```python
from build123d import *

# Parameters (mm, degrees)
F0_W      = 124.8
F0_H      = 81
F1_DEPTH  = 15.39
F2_W      = 120.8
F2_H      = 77
F3_DEPTH  = 13.39
F4_W      = 124.8
F4_H      = 3
F5_DEPTH  = 1.15
F6_W      = 124.8
F6_H      = 3
F7_DEPTH  = 1.15
F8_W      = 78.7
F8_H      = 3
F9_DEPTH  = 1.15
F10_W     = 78.7
F10_H     = 3
F11_DEPTH = 1.15
F12_W     = 10
F12_H     = 10
F13_DEPTH = 11.82
F14_W     = 10
F14_H     = 10
F15_DEPTH = 11.82
F16_W     = 10
F16_H     = 10
F17_DEPTH = 11.82
F18_W     = 10
F18_H     = 10
F19_DEPTH = 11.82
F20_R     = 1.5
F21_DEPTH = 11.82
F22_R     = 1.5
F23_DEPTH = 11.82
F24_R     = 1.5
F25_DEPTH = 11.82
F26_R     = 1.5
F27_DEPTH = 11.82
F28_W     = 26
F28_H     = 45
F29_DEPTH = 2.001
F30_W     = 12.8
F30_H     = 30.7
F31_DEPTH = 2.001
F32_W     = 17
F32_H     = 12.8
F33_DEPTH = 2.001
F34_R     = 3
F35_DEPTH = 3.3


with BuildPart() as f1:
    # F0 (on Top) → F1 (new body)
    with BuildSketch(Plane.XY):
        Rectangle(F0_W, F0_H)
    extrude(amount=F1_DEPTH)

    # F2 (on face) → F3 (cut)
    with BuildSketch(Plane.XY.offset(15.39)):
        Rectangle(F2_W, F2_H)
    extrude(amount=-F3_DEPTH, mode=Mode.SUBTRACT)

    # F4 (on face) → F5 (cut)
    with BuildSketch(Plane(origin=(0, 40.5, 0), x_dir=(-1, 0, 0), z_dir=(0, 1, 0))):
        with Locations((0, 13.89)):
            Rectangle(F4_W, F4_H)
    extrude(amount=-F5_DEPTH, mode=Mode.SUBTRACT)

    # F6 (on face) → F7 (cut)
    with BuildSketch(Plane.XZ.offset(40.5)):
        with Locations((0, 13.89)):
            Rectangle(F6_W, F6_H)
    extrude(amount=-F7_DEPTH, mode=Mode.SUBTRACT)

    # F8 (on face) → F9 (cut)
    with BuildSketch(Plane(origin=(-62.4, 0, 0), x_dir=(0, -1, 0), z_dir=(-1, 0, 0))):
        with Locations((0, 13.89)):
            Rectangle(F8_W, F8_H)
    extrude(amount=-F9_DEPTH, mode=Mode.SUBTRACT)

    # F10 (on face) → F11 (cut)
    with BuildSketch(Plane.YZ.offset(62.4)):
        with Locations((0, 13.89)):
            Rectangle(F10_W, F10_H)
    extrude(amount=-F11_DEPTH, mode=Mode.SUBTRACT)

    # F12 (on face) → F13 (join)
    with BuildSketch(Plane.XY.offset(2)):
        with Locations((-55.4, 33.5)):
            Rectangle(F12_W, F12_H)
    extrude(amount=F13_DEPTH)

    # F14 (on face) → F15 (join)
    with BuildSketch(Plane.XY.offset(2)):
        with Locations((-55.4, -33.5)):
            Rectangle(F14_W, F14_H)
    extrude(amount=F15_DEPTH)

    # F16 (on face) → F17 (join)
    with BuildSketch(Plane.XY.offset(2)):
        with Locations((55.4, -33.5)):
            Rectangle(F16_W, F16_H)
    extrude(amount=F17_DEPTH)

    # F18 (on face) → F19 (join)
    with BuildSketch(Plane.XY.offset(2)):
        with Locations((55.4, 33.5)):
            Rectangle(F18_W, F18_H)
    extrude(amount=F19_DEPTH)

    # F20 (on face) → F21 (cut)
    with BuildSketch(Plane.XY.offset(13.82)):
        with Locations((-55, 33.5)):
            Circle(F20_R)
    extrude(amount=-F21_DEPTH, mode=Mode.SUBTRACT)

    # F22 (on face) → F23 (cut)
    with BuildSketch(Plane.XY.offset(13.82)):
        with Locations((-55, -33.5)):
            Circle(F22_R)
    extrude(amount=-F23_DEPTH, mode=Mode.SUBTRACT)

    # F24 (on face) → F25 (cut)
    with BuildSketch(Plane.XY.offset(13.82)):
        with Locations((55, -33.5)):
            Circle(F24_R)
    extrude(amount=-F25_DEPTH, mode=Mode.SUBTRACT)

    # F26 (on face) → F27 (cut)
    with BuildSketch(Plane.XY.offset(13.82)):
        with Locations((55, 33.5)):
            Circle(F26_R)
    extrude(amount=-F27_DEPTH, mode=Mode.SUBTRACT)

    # F28 (on face) → F29 (cut, through all)
    with BuildSketch(Plane.XY.offset(2)):
        with Locations((44.4, 5)):
            Rectangle(F28_W, F28_H)
    extrude(amount=-F29_DEPTH, mode=Mode.SUBTRACT)

    # F30 (on face) → F31 (cut, through all)
    with BuildSketch(Plane.XY.offset(2)):
        with Locations((9.5, 0)):
            Rectangle(F30_W, F30_H)
    extrude(amount=-F31_DEPTH, mode=Mode.SUBTRACT)

    # F32 (on face) → F33 (cut, through all)
    with BuildSketch(Plane.XY.offset(2)):
        with Locations((24.9, -29.1)):
            Rectangle(F32_W, F32_H)
    extrude(amount=-F33_DEPTH, mode=Mode.SUBTRACT)

    # F34 (on face) → F35 (join)
    with BuildSketch(Plane.XY.offset(2)):
        with Locations((24.4, 13.2)):
            Circle(F34_R)
        with Locations((24.4, -15.8)):
            Circle(F34_R)
        with Locations((-34.6, 13.2)):
            Circle(F34_R)
        with Locations((-34.6, -15.8)):
            Circle(F34_R)
    extrude(amount=F35_DEPTH)


solid = f1.part
```
Source: CAD feature listing. Evaluate the final solid. Frame: model axes, mm. A direction names the side the tool comes from. Round coordinates to 2 decimals unless told otherwise and drop trailing zeros. Loops run counter-clockwise (first coordinate to the right, second up) from the corner with the lowest first, then second, coordinate; pieces in that order, holes last.
(1) Section query D-D (y = -3). Output: boundary loops of the cut face in (x, z).
From the geometry:
outline: (-62.4, 0) - (3.1, 0) - (3.1, 2) - (-60.4, 2) - (-60.4, 15.39) - (-61.25, 15.39) - (-61.25, 12.39) - (-62.4, 12.39) - close; (15.9, 0) - (31.4, 0) - (31.4, 2) - (15.9, 2) - close; (57.4, 0) - (62.4, 0) - (62.4, 12.39) - (61.25, 12.39) - (61.25, 15.39) - (60.4, 15.39) - (60.4, 2) - (57.4, 2) - close
(2) Pull-direction query (Y, two-part tool) for faces 3 (the flat face through (1, 39.35, 14)), 4 (the flat face through (56, -32, 13.82)), 5 (the flat face through (61.25, -1, 14)); classes: +Y half, -Y half, draft (parallel to the pull), parting line (faces both ways), or undercut.
From the geometry:
face 3: +Y half
face 4: undercut
face 5: draft
(3) Section query C-C (z = 9). Output: boundary loops of the cut face in (x, y), and give its area (3 significant figures).
From the geometry:
outline: (-62.4, -40.5) - (62.4, -40.5) - (62.4, 40.5) - (-62.4, 40.5) - close; hole (-60.4, -28.5) - (-50.4, -28.5) - (-50.4, -38.5) - (50.4, -38.5) - (50.4, -28.5) - (60.4, -28.5) - (60.4, 28.5) - (50.4, 28.5) - (50.4, 38.5) - (-50.4, 38.5) - (-50.4, 28.5) - (-60.4, 28.5) - close; hole circle Ø3 at (-55, -33.5); hole circle Ø3 at (-55, 33.5); hole circle Ø3 at (55, -33.5); hole circle Ø3 at (55, 33.5)
area: 1,180 mm2
(4) Section query A-A (y = 21). Output: boundary loops of the cut face in (x, z).
From the geometry:
outline: (-62.4, 0) - (31.4, 0) - (31.4, 2) - (-60.4, 2) - (-60.4, 15.39) - (-61.25, 15.39) - (-61.25, 12.39) - (-62.4, 12.39) - close; (57.4, 0) - (62.4, 0) - (62.4, 12.39) - (61.25, 12.39) - (61.25, 15.39) - (60.4, 15.39) - (60.4, 2) - (57.4, 2) - close
(5) Contact query for flat-ended pins moving along their axis: pin 1 Ø2.5 at (x, y) = (55, -33.5) entering from +Z; pin 2 Ø3 at (x, y) = (-35, 13.5) entering from +Z; pin 3 Ø4 at (x, y) = (-55, 33.5) entering from +Z. Output: stop coordinate, or through.
From the geometry:
pin 1: stops at z = 2
pin 2: stops at z = 5.3
pin 3: stops at z = 13.82
(6) Material intervals for probe 1 along Y at (x, z) = (-55, 11); probe 2 along Y at (x, z) = (21.5, 14.25); probe 3 along X at (y, z) = (-33, 7.25), sorted ascending.
From the geometry:
probe 1: y = -40.5 to -35, -32 to -28.5, 28.5 to 32, 35 to 40.5
probe 2: y = -39.35 to -38.5, 38.5 to 39.35
probe 3: x = -62.4 to -56.41, -53.59 to -50.4, 50.4 to 53.59, 56.41 to 62.4
(7) Section query B-B (x = 55). Output: boundary loops of the cut face in (y, z).
From the geometry:
outline: (-40.5, 0) - (-17.5, 0) - (-17.5, 2) - (-28.5, 2) - (-28.5, 13.82) - (-32, 13.82) - (-32, 2) - (-35, 2) - (-35, 13.82) - (-38.5, 13.82) - (-38.5, 15.39) - (-39.35, 15.39) - (-39.35, 12.39) - (-40.5, 12.39) - close; (27.5, 0) - (40.5, 0) - (40.5, 12.39) - (39.35, 12.39) - (39.35, 15.39) - (38.5, 15.39) - (38.5, 13.82) - (35, 13.82) - (35, 2) - (32, 2) - (32, 13.82) - (28.5, 13.82) - (28.5, 2) - (27.5, 2) - close
(8) Access query for faces 1 (the flat face through (-15, 1, 0)), 2 (the flat face through (56, 35, 13.82)). Directions: +Z, -Z, +X, -X, +Y, -Y. A direction counts if a zero-diameter tool reaches every point of the face in a straight line with its end or side. Return the directions, or none.
From the geometry:
face 1: -Z, +X, -X, +Y, -Y
face 2: +Z
